Autodesk Inventor part; units mm, degrees
ref_plane "Work Plane2" through (0, 0, 13.75) normal (0, 0, 1) x (1, 0, 0)
ref_plane "YZ Plane" through (0, 0, 0) normal (1, 0, 0) x (0, 1, 0)
ref_plane "XZ Plane" through (0, 0, 0) normal (0, 1, 0) x (-1, 0, 0)
sketch "Sketch1" plane through (0, 0, 0) normal (0, 0, 1) x (1, 0, 0)
  circle A0 centre (0, 0) radius 24
  circle A1 centre (0, 0) radius 22.7
  dimension "d0" = 48
  dimension "d1" = 45.4
extrude "Extrusion1" add sketch "Sketch1" along normal blind 5
sketch "Sketch2" plane through (0, 0, 0) normal (0, 0, -1) x (-1, 0, 0)
  circle A0 centre (0, 0) radius 24
  circle A1 centre (0, 0) radius 7.5
  dimension "d4" = 15
extrude "Extrusion2" add sketch "Sketch2" along normal blind 5
sketch "Sketch3" plane through (0, 0, 5) normal (0, 0, 1) x (1, 0, 0)
  circle A0 centre (0, 0) radius 22.7
  circle A1 centre (0, 0) radius 24
  arc A2 (8.8209, 21.2954) -> (-8.8209, 21.2954) centre (0, 0) ccw
  arc A3 (9.0505, 21.8498) -> (-9.0505, 21.8498) centre (0, 0) ccw
  circle A4 centre (0, 0) radius 7.5
  line L0 (0, 0) -> (0, 19.001)
  line L1 (-8.8209, 21.2954) -> (-9.0505, 21.8498)
  line L2 (8.8209, 21.2954) -> (9.0505, 21.8498)
  arc A5 (-21.2954, 8.8209) -> (-21.2954, -8.8209) centre (0, 0) ccw
  arc A6 (-21.8498, 9.0505) -> (-21.8498, -9.0505) centre (0, 0) ccw
  line L3 (-21.2954, -8.8209) -> (-21.8498, -9.0505)
  line L4 (-21.2954, 8.8209) -> (-21.8498, 9.0505)
  arc A7 (-8.8209, -21.2954) -> (8.8209, -21.2954) centre (0, 0) ccw
  arc A8 (-9.0505, -21.8498) -> (9.0505, -21.8498) centre (0, 0) ccw
  line L5 (8.8209, -21.2954) -> (9.0505, -21.8498)
  line L6 (-8.8209, -21.2954) -> (-9.0505, -21.8498)
  arc A9 (21.2954, -8.8209) -> (21.2954, 8.8209) centre (0, 0) ccw
  arc A10 (21.8498, -9.0505) -> (21.8498, 9.0505) centre (0, 0) ccw
  line L7 (21.2954, 8.8209) -> (21.8498, 9.0505)
  line L8 (21.2954, -8.8209) -> (21.8498, -9.0505)
  point P0 (-19.001, 0)
  point P1 (0, -19.001)
  point P2 (19.001, 0)
  dimension "d7" = 0.35
  dimension "d8" = 0.35
  dimension "d13" = 360
extrude "Extrusion3" add sketch "Sketch3" along normal blind 10 contours A2 L1 A3 L2 | A5 L3 A6 L4 | A7 L5 A8 L6 | A9 L7 A10 L8
ref_plane "Work Plane2" through (0, 0, 13.75) normal (0, 0, 1) x (1, 0, 0)
sketch "Sketch6" plane through (0, 0, 13.75) normal (0, 0, 1) x (1, 0, 0)
  arc A0 (-8.8209, -21.2954) -> (8.8209, -21.2954) centre (0, 0) ccw
  arc A1 (-8.7252, -21.0645) -> (8.7252, -21.0645) centre (0, 0) ccw
  line L0 (-8.7252, -21.0645) -> (-8.8209, -21.2954)
  line L1 (8.7252, -21.0645) -> (8.8209, -21.2954)
  dimension "d19" = 0.25
extrude "Extrusion4" add sketch "Sketch6" along normal mid plane 0.5
pattern_circular "Circular Pattern1" count 4 over 360 about axis through (0, 0, -10) along (0, 0, 1) of "Extrusion4"
sketch "Sketch7" plane through (0, 0, -5) normal (0, 0, -1) x (-1, 0, 0)
  circle A0 centre (0, 0) radius 7.5
  circle A1 centre (0, 0) radius 29
  circle A2 centre (0, 0) radius 24
  dimension "d26" = 58
extrude "Extrusion5" add sketch "Sketch7" against normal blind 10 contours A1
sketch "Sketch8" plane through (0, 0, -5) normal (0, 0, -1) x (-1, 0, 0)
  circle A0 centre (17.9207, 17.9207) radius 1.425
  circle A1 centre (17.9207, -17.9207) radius 1.425
  circle A2 centre (-17.9207, -17.9207) radius 1.425
  circle A3 centre (-17.9207, 17.9207) radius 1.425
  point P0 (0, 0)
  point P1 (0, 0)
hole "Hole1" at (17.9207, 17.9207, -5) at (17.9207, -17.9207, -5) at (-17.9207, -17.9207, -5) at (-17.9207, 17.9207, -5) direction (0, 0, 1) diameter 2.459 depth 8.8 counterbore diameter 6 counterbore depth 2
equation "\"d10\" = 0.5 * d9"
properties part number "Housing of planetary gearbox" material "Steel, Alloy"
The listing builds one solid part. Answer for the finished solid, in the listing's coordinates (mm). A direction names the side the tool comes from. Give positions to 0.01 mm unless a question says otherwise; leave off trailing zeros. Loops run counter-clockwise (first coordinate to the right, second up) from the corner with the lowest first, then second, coordinate; pieces in that order, holes last. Notation, with made-up numbers: (-20.5, 12) - (-15.5, 12) arc R11 ccw to (-15.5, 22) - close; hole circle Ø6 at (-27.75, -12.75). An arc over 180 degrees is marked (long way). Answer as a JSON object with one key per item and string values.
1. A cutting plane is placed at A-A (x = 0). Write down the section's boundary in (y, z), then the cut area to 3 significant figures.
Determined:
{"outline": "(-29, -5) - (-7.5, -5) - (-7.5, 0) - (-22.7, 0) - (-22.7, 5) - (-23.05, 5) - (-23.05, 13.5) - (-22.8, 13.5) - (-22.8, 14) - (-23.05, 14) - (-23.05, 15) - (-23.65, 15) - (-23.65, 5) - (-29, 5) - close; (7.5, -5) - (29, -5) - (29, 5) - (23.65, 5) - (23.65, 15) - (23.05, 15) - (23.05, 14) - (22.8, 14) - (22.8, 13.5) - (23.05, 13.5) - (23.05, 5) - (22.7, 5) - (22.7, 0) - (7.5, 0) - close", "area": "290 mm²"}
2. For faces 1 (the cylindrical face through (17.55, -16.75, 0.45)), 2 (the cylindrical face through (22.8, 0.1, 13.7)), 3 (the cylindrical face through (0.13, -23.65, 9.93)), 4 (the cylindrical face through (0.13, -23.05, 9.19)), determine the directions among +Z, -Z, +X, -X, +Y, -Y from which every point of the face is accessible in a straight line to the end or side of a thin tool.
Determined:
{"face 1": "-Z", "face 2": "+Z", "face 3": "+Z, -Y", "face 4": "none"}
3. For a pull along X with two mould halves and no side action, classify faces 5 (the cylindrical face through (-0.13, 23.65, 9.93)), 6 (the flat face through (0, -23.2, 15)), 7 (the cylindrical face through (7.493, -0.33, -2.465)), 8 (the cylindrical face through (-0.1, 22.8, 13.7)) as pulls with the +X half, pulls with the -X half, needs draft (parallel to the pull), parting line crosses it, or undercut.
Determined:
{"face 5": "parting line crosses it", "face 6": "needs draft", "face 7": "undercut", "face 8": "undercut"}
4. A cutting plane is placed at C-C (x = 12.5). Write down the section's boundary in (y, z), then the cut area to 3 significant figures.
Determined:
{"outline": "(-26.17, -5) - (26.17, -5) - (26.17, 5) - (18.95, 5) - (18.95, 0) - (-18.95, 0) - (-18.95, 5) - (-26.17, 5) - close", "area": "334 mm²"}
5. A cutting plane is placed at D-D (y = 17.5). Write down the section's boundary in (x, z).
Determined:
{"outline": "(-23.12, -5) - (-20.89, -5) - (-20.89, -3) - (-19.08, -3) - (-19.08, 3.8) - (-16.77, 3.8) - (-16.77, -3) - (-14.95, -3) - (-14.95, -5) - (14.95, -5) - (14.95, -3) - (16.77, -3) - (16.77, 3.8) - (19.08, 3.8) - (19.08, -3) - (20.89, -3) - (20.89, -5) - (23.12, -5) - (23.12, 5) - (14.46, 5) - (14.46, 0) - (-14.46, 0) - (-14.46, 5) - (-23.12, 5) - close"}
6. Find the intervals of material crossed by L1, parallel to X at y = 0, z = 10.5; L2, parallel to Y at x = 0, z = -2.3; L3, parallel to X at y = -18.5, z = -0.25, in increasing order. Write a range as [from, to].
Determined:
{"L1": "[-23.65, -23.05], [23.05, 23.65]", "L2": "[-29, -7.5], [7.5, 29]", "L3": "[-22.33, -19.01], [-16.84, 16.84], [19.01, 22.33]"}
7. Flat-ended cylindrical pins translate along their axes: pin 1 Ø3 at (x, y) = (17.5, 19) entering from -Z; pin 2 Ø5.5 at (x, y) = (17.92, 17.92) entering from +Z; pin 3 Ø8 at (y, z) = (-19.5, 6) entering from -X; pin 4 Ø5 at (x, z) = (18.5, 9.5) entering from -Y. Find the tip coordinate at first contact, or state that the pin passes through.
Determined:
{"pin 1": "z = -3", "pin 2": "z = 5", "pin 3": "x = -24.43", "pin 4": "through"}
